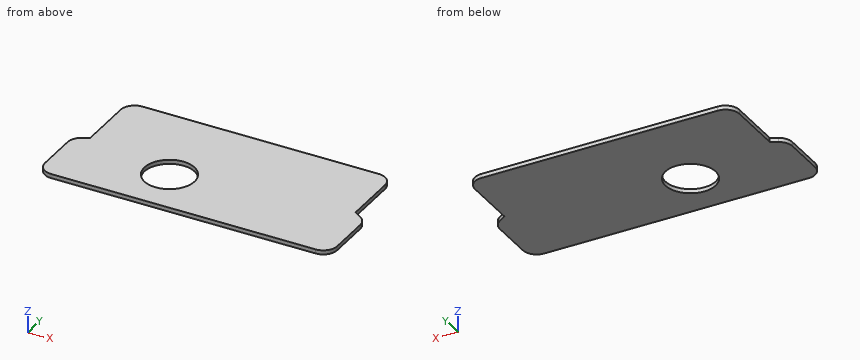
```python
from build123d import *

# Parameters (mm, degrees)
SKETCH_1_R      = 18
EXTRUDE_1_DEPTH = 3


with BuildPart() as part:
    # 草图1 → 凸台-拉伸1 (new body)
    with BuildSketch(Plane.XY):
        with BuildLine():
            Line((0, 10), (0, 39.186569494))
            ThreePointArc((0, 39.186569494), (1.375838219, 44.248568464), (5.124766715, 47.917669105))
            Line((5.124766715, 47.917669105), (10, 50.639880584))
            Line((10, 50.639880584), (10, 90))
            ThreePointArc((10, 90), (12.928932188, 97.071067812), (20, 100))
            Line((20, 100), (190, 100))
            ThreePointArc((190, 100), (197.071067812, 97.071067812), (200, 90))
            Line((200, 90), (200, 51.963395008))
            Line((200, 51.963395008), (205.683304945, 48.037782396))
            ThreePointArc((205.683304945, 48.037782396), (208.855310538, 44.455580593), (210, 39.809778695))
            Line((210, 39.809778695), (210, 10))
            ThreePointArc((210, 10), (207.071067812, 2.928932188), (200, 0))
            Line((200, 0), (10, 0))
            ThreePointArc((10, 0), (2.928932188, 2.928932188), (0, 10))
        make_face()
        with Locations((75.264593403, 35.622477185)):
            Circle(SKETCH_1_R, mode=Mode.SUBTRACT)
    extrude(amount=EXTRUDE_1_DEPTH)


solid = part.part
```
Build history of the part. All positions in model axes, mm. Give positions to 0.01 mm unless a question says otherwise; leave off trailing zeros. Loops run counter-clockwise (first coordinate to the right, second up) from the corner with the lowest first, then second, coordinate; pieces in that order, holes last.
1) Band-saw the part on C-C on z = 1.45. List the corners of the cut face in (x, y).
Values follow:
outline: (0, 10) arc R10 ccw to (10, 0) - (200, 0) arc R10 ccw to (210, 10) - (210, 39.81) arc R10 ccw to (205.68, 48.04) - (200, 51.96) - (200, 90) arc R10 ccw to (190, 100) - (20, 100) arc R10 ccw to (10, 90) - (10, 50.64) - (5.12, 47.92) arc R10 ccw to (0, 39.19) - close; hole circle Ø36 at (75.26, 35.62)
2) Band-saw the part on D-D on y = 86.5. List the corners of the cut face in (x, z), then the cut area to 3 significant figures.
Values follow:
outline: (10, 0) - (200, 0) - (200, 3) - (10, 3) - close
area: 570 mm2
3) Probe line 1 along Y through (x, z) = (74.5, 1.3); line 2 along Y through (x, z) = (67, 0.3); line 3 along X through (y, z) = (22, 0.3). List the from-to ranges inside material, lowest first.
Values follow:
line 1: y = 0 to 17.64, 53.61 to 100
line 2: y = 0 to 19.63, 51.61 to 100
line 3: x = 0 to 63.5, 87.03 to 210
4) Band-saw the part on A-A on x = 80.5. List the corners of the cut face in (y, z), then the cut area to 3 significant figures.
Values follow:
outline: (0, 0) - (18.4, 0) - (18.4, 3) - (0, 3) - close; (52.84, 0) - (100, 0) - (100, 3) - (52.84, 3) - close
area: 197 mm2
5) Drop flat-ended pins along their axis: P1, Ø1.5, axis at y = 84.5, z = 1, coming from the -X side; P2, Ø0.9, axis at y = 67, z = 1.5, coming from the +X side. Give the stop position or say it passes through.
Values follow:
P1: stops at x = 10
P2: stops at x = 200
6) Band-saw the part on B-B on y = 22. List the corners of the cut face in (x, z), then the cut area to 3 significant figures.
Values follow:
outline: (0, 0) - (63.5, 0) - (63.5, 3) - (0, 3) - close; (87.03, 0) - (210, 0) - (210, 3) - (87.03, 3) - close
area: 559 mm2
